Geometry check sheet. Reference: the model listing, model coordinates, mm. A direction names the side the tool comes from. Coordinates: 2 decimals unless noted, no trailing zeros. Loops run counter-clockwise (first coordinate to the right, second up) from the corner with the lowest first, then second, coordinate; pieces in that order, holes last. Notation, with made-up numbers: (87.5, 86) - (98.5, 86) arc R7 cw to (98.5, 92) - close; hole circle Ø6 at (54.25, 48). An arc over 180 degrees is marked (long way). Write each question's results on one line, items separated by ' | '. Start each with the question number.
(1) Mould release check, pull along Z, two halves, no side actions. Record for faces 1 (the face through (11.8, 10, -18)), 2 (the face through (6, 10, 0)), 3 (the face through (5.944, 21.287, -36.259)), 4 (the face through (11.4, 21.43, -18.73)): pulls with the +Z half, pulls with the -Z half, needs draft (parallel to the pull), parting line crosses it, or undercut.
(2) Material ranges on probe 1 along X at (y, z) = (11.75, -3.5); probe 2 along Z at (x, y) = (2.5, 14.5); probe 3 along Y at (x, z) = (8.25, -20), recorded low to high.
(3) Go/stop test with a flat-tipped pin: pin 1 Ø1 at (x, z) = (9, -4) entering from -Y. Record where the tip stops, or that it passes through.
(4) Sectioned sample at A-A (y = 12.5). Enter the section's corners in (x, z).
(5) Sectioned sample at C-C (z = -19). Enter the section's corners in (x, y), plus the area to 3 significant figures.
(6) Access from +Z, -Z, +X, -X, +Y, -Y to the whole of each face (thin tool, end or side, straight path). Record for faces 5 (the face through (0.2, 10, -19)), 6 (the face through (0, 10, -19)).
(7) Sectioned sample at B-B (x = 6). Enter the section's corners in (y, z).
Autodesk Inventor part; units mm, degrees
ref_plane "YZ Plane" through (0, 0, 0) normal (1, 0, 0) x (0, 1, 0)
ref_plane "XZ Plane" through (0, 0, 0) normal (0, 1, 0) x (-1, 0, 0)
ref_plane "XY Plane" through (0, 0, 0) normal (0, 0, 1) x (1, 0, 0)
sketch "Sketch1" plane through (0, 0, 0) normal (0, 1, 0) x (-1, 0, 0)
  line L0 (0, 0) -> (-12, 0)
  line L1 (-12, 0) -> (-12, -37)
  line L2 (-12, -37) -> (0, -37)
  line L3 (0, -37) -> (0, 0)
  dimension "d0" = 12
  dimension "d1" = 37
extrude "Extrusion1" add sketch "Sketch1" along normal blind 22
fillet "Fillet1" radius 2 8 edges at (6, 22, -37) (0, 22, -18.5) (12, 22, -18.5) (6, 22, 0) (0, 11, 0) (0, 11, -37) (12, 11, -37) (12, 11, 0)
shell "Shell1" thickness 0.2 removed faces 1 at (8, 0, -13)
sketch "Sketch2" plane through (2, 0, 0) normal (0, 0, 1) x (1, 0, 0)
  line L0 (8, 0) -> (0, 0)
  line L1 (8, 0) -> (8, 20)
  line L2 (0, 0) -> (8, 0)
  line L3 (8, 0) -> (8, 1)
  line L4 (8, 1) -> (0, 1)
  line L5 (0, 1) -> (0, 0)
  point P0 (-2, 0)
  dimension "d6" = 1
extrude "Extrusion2" cut sketch "Sketch2" against normal blind 22
properties part number "Top_Case"
Outcome:
1) face 1: undercut | face 2: pulls with the +Z half | face 3: undercut | face 4: needs draft
2) probe 1: x = 0 to 0.2, 11.8 to 12 | probe 2: z = -37 to -36.8, -0.2 to 0 | probe 3: y = 21.8 to 22
3) pin 1: stops at y = 21.8
4) outline: (0, -35) arc R2 ccw to (2, -37) - (10, -37) arc R2 ccw to (12, -35) - (12, -2) arc R2 ccw to (10, 0) - (2, 0) arc R2 ccw to (0, -2) - close; hole (0.2, -35) arc R1.8 ccw to (2, -36.8) - (10, -36.8) arc R1.8 ccw to (11.8, -35) - (11.8, -2) arc R1.8 ccw to (10, -0.2) - (2, -0.2) arc R1.8 ccw to (0.2, -2) - close
5) outline: (0, 0) - (0.2, 0) - (0.2, 20) arc R1.8 cw to (2, 21.8) - (10, 21.8) arc R1.8 cw to (11.8, 20) - (11.8, 0) - (12, 0) - (12, 20) arc R2 ccw to (10, 22) - (2, 22) arc R2 ccw to (0, 20) - close | area: 10.8 mm2
6) face 5: -Y | face 6: +Z, -Z, -X, +Y, -Y
7) outline: (0, -37) - (20, -37) arc R2 ccw to (22, -35) - (22, -2) arc R2 ccw to (20, 0) - (1, 0) - (1, -0.2) - (20, -0.2) arc R1.8 cw to (21.8, -2) - (21.8, -35) arc R1.8 cw to (20, -36.8) - (0, -36.8) - close
